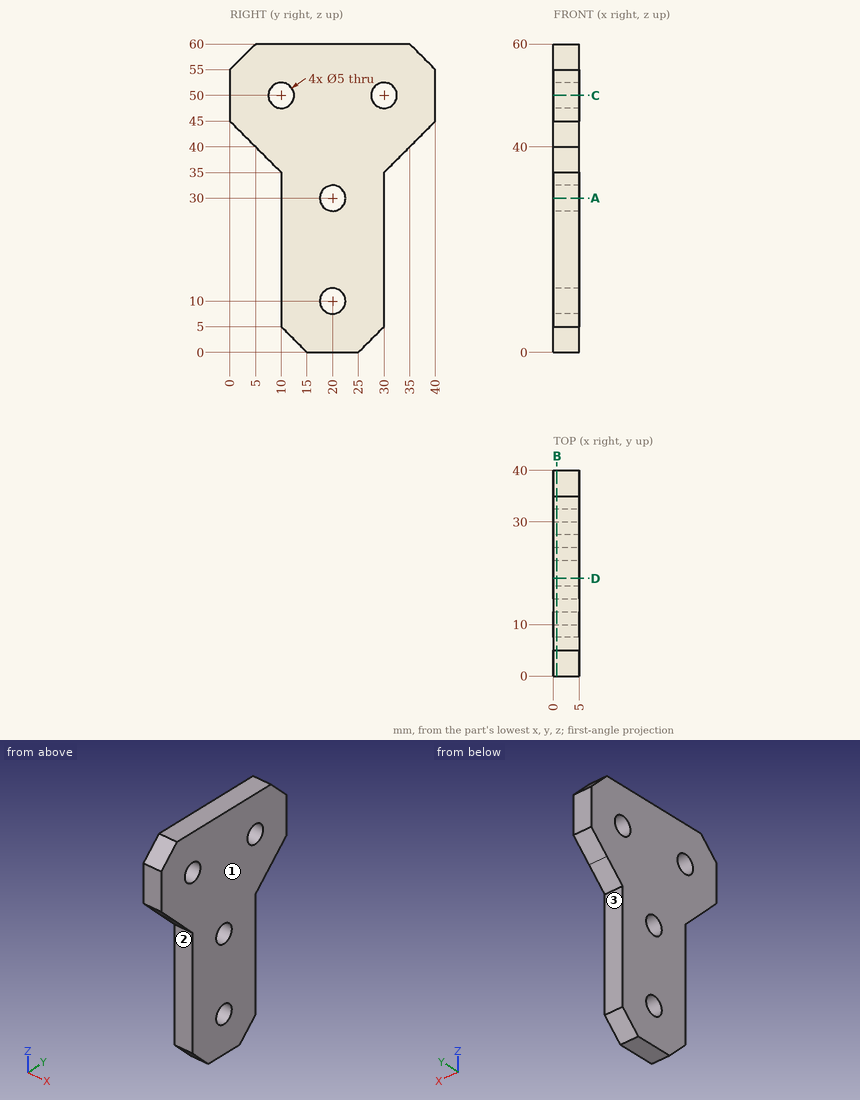
Here's the drawing with two shaded views (mm, measured from the low corner). I have some questions. A direction names the side the tool comes from. Coordinates: 2 decimals unless noted, no trailing zeros. Write each loop counter-clockwise with the first axis right and the second up, starting at its lowest first coordinate (ties: lowest second). Pieces come first, ordered by that corner, then holes. Notation, with made-up numbers: M 88,81.5 L 95,81.5 A35 ccw 95,114.5 Z; hole C 64,-36 d9. An arc over 180 degrees is marked long. Answer as CSV lines item,"result". Start each with the question number.
1) I want a section at D-D, the plane y = 19. Please give me the cut outline in (x, z).
2) I want a section at C-C, the plane z = 50. Please give me the cut outline in (x, y), and give its area (3 significant figures).
3) For P1, Ø1.5, axis at x = 0.5, y = 35, coming from the -Z side; P2, Ø1.5, axis at x = 1.5, z = 17, coming from the -Y side; P3, Ø1.5, axis at x = 3.5, z = 36.5, coming from the -Y side, each with a flat end and sliding along its axis, tell me the tip position at first contact or that it passes through.
4) Please list where these lines run through material, in increasing order: line 1 (Z direction, x = 1.55, y = 20); line 2 (Y direction, x = 2.25, z = 20); line 3 (Z direction, x = 1.2, y = 21). Write a range as from..to.
5) I want a section at A-A, the plane z = 30. Please give me the cut outline in (x, y).
6) I want a section at B-B, the plane x = 0.65. Give the number of separate pieces and of enclosed holes in the cut face, and give its area (3 significant figures).
7) For the marked faces 1, 2 and 3, which set-ups out of +Z, -Z, +X, -X, +Y, -Y let a thin tool reach every point of the face, with its end or its side?
Data:
1,outline,"M 0,0 L 5,0 L 5,7.71 L 0,7.71 Z; M 0,12.29 L 5,12.29 L 5,27.71 L 0,27.71 Z; M 0,32.29 L 5,32.29 L 5,60 L 0,60 Z"
2,outline,"M 0,0 L 5,0 L 5,7.5 L 0,7.5 Z; M 0,12.5 L 5,12.5 L 5,27.5 L 0,27.5 Z; M 0,32.5 L 5,32.5 L 5,40 L 0,40 Z"
2,area,"150 mm^2"
3,P1,"stops at z = 39.25"
3,P2,"stops at y = 10"
3,P3,"stops at y = 7.75"
4,line 1,"z = 0..7.5, 12.5..27.5, 32.5..60"
4,line 2,"y = 10..30"
4,line 3,"z = 0..7.71, 12.29..27.71, 32.29..60"
5,outline,"M 0,10 L 5,10 L 5,17.5 L 0,17.5 Z; M 0,22.5 L 5,22.5 L 5,30 L 0,30 Z"
6,separate pieces,"1"
6,enclosed holes,"4"
6,area,"1,470 mm^2"
7,face 1,"+Z, -Z, +X, +Y, -Y"
7,face 2,"-Z, +X, -X, -Y"
7,face 3,"-Z, +X, -X, +Y"
